Autodesk Inventor part; units mm, degrees
ref_plane "YZ Plane" through (0, 0, 0) normal (1, 0, 0) x (0, 1, 0)
ref_plane "XZ Plane" through (0, 0, 0) normal (0, 1, 0) x (-1, 0, 0)
ref_plane "XY Plane" through (0, 0, 0) normal (0, 0, 1) x (1, 0, 0)
sketch "Sketch1" plane through (0, 0, 0) normal (0, 0, 1) x (1, 0, 0)
  line L0 (0, 0) -> (25.7, 0)
  line L1 (25.7, 0) -> (25.7, 44.3)
  line L2 (25.7, 44.3) -> (0, 44.3)
  line L3 (0, 44.3) -> (0, 0)
  dimension "d0" = 25.7
  dimension "d1" = 44.3
extrude "Extrusion1" add sketch "Sketch1" along normal blind 16.6
sketch "Sketch2" plane through (0, 44.3, 0) normal (0, 1, 0) x (1, 0, 0)
  line L0 (0, 0) -> (0, -16.6)
  circle A0 centre (6.15, -8.3) radius 4.15
  circle A1 centre (19.55, -8.3) radius 2.85
  dimension "d4" = 8.3
  dimension "d5" = 5.7
  dimension "d6" = 13.4
  dimension "d7" = 6.15
extrude "Extrusion2" add sketch "Sketch2" along normal blind 3.3
sketch "Sketch3" plane through (6.15, 47.6, 8.3) normal (0, 1, 0) x (1, 0, 0)
  circle A0 centre (0, 0) radius 4.15
  circle A1 centre (0, 0) radius 2.85
  point P0 (-6.15, 8.3)
  dimension "d10" = 5.7
extrude "Extrusion3" cut sketch "Sketch3" against normal blind 3 contours A1
fillet "Fillet1" radius 3 4 edges at (25.7, 22.15, 16.6) (25.7, 22.15, 0) (0, 22.15, 16.6) (0, 22.15, 0)
fillet "Fillet2" radius 1 16 edges at (12.85, 44.3, 16.6) (24.8213, 44.3, 15.7213) (25.7, 44.3, 8.3) (24.8213, 44.3, 0.8787) (12.85, 44.3, 0) (0.8787, 44.3, 0.8787) (0, 44.3, 8.3) (0.8787, 44.3, 15.7213) (12.85, 0, 16.6) (0.8787, 0, 15.7213) (0, 0, 8.3) (0.8787, 0, 0.8787) (12.85, 0, 0) (24.8213, 0, 0.8787) (25.7, 0, 8.3) (24.8213, 0, 15.7213)
properties part number "Battery9V"
Can you work these out from the model? Positions are in its coordinate system, mm. A direction names the side the tool comes from. Coordinates: 2 decimals unless noted, no trailing zeros. Order: outer loops, then holes, each group sorted by start corner. A loop starts at its lowest first (then second) coordinate and runs counter-clockwise, first axis right, second up.
1. If we section it at C-C (z = 8.3): Please give me the cut outline in (x, y), then the cut area to 3 significant figures.
2. Thinking about a two-plate mould opening in X: for faces 1 (the face through (25.415, 43.999, 8.374)), 2 (the face through (12.712, 0.301, 0.285)), 3 (the face through (13, 44.3, 8)), which applies, +X half, -X half, draft (parallel to the pull), parting line (faces both ways), or undercut?
3. For faces 4 (the face through (0.285, 0.301, 8.374)), 5 (the face through (5.779, 46.121, 5.474)), which set-ups out of +Z, -Z, +X, -X, +Y, -Y let a thin tool reach every point of the face, with its end or its side?
4. If we section it at B-B (y = 42): Please give me the cut outline in (x, z), then the cut area to 3 significant figures.
5. If we section it at D-D (x = 6.15): Please give me the cut outline in (y, z).
6. I need wall thicknesses on line 1 (X direction, y = 45.5, z = 8.3); line 2 (Z direction, x = 6.15, y = 46.2); line 3 (Y direction, x = 21, z = 15.5). Which ranges of each line are inside material? Lowest first, please.
7. If we section it at A-A (x = 19.55): Please give me the cut outline in (y, z).
Entries:
1. outline: (0, 1) arc R1 ccw to (1, 0) - (24.7, 0) arc R1 ccw to (25.7, 1) - (25.7, 43.3) arc R1 ccw to (24.7, 44.3) - (22.4, 44.3) - (22.4, 47.6) - (16.7, 47.6) - (16.7, 44.3) - (10.3, 44.3) - (10.3, 47.6) - (9, 47.6) - (9, 44.6) - (3.3, 44.6) - (3.3, 47.6) - (2, 47.6) - (2, 44.3) - (1, 44.3) arc R1 ccw to (0, 43.3) - close
1. area: 1,170 mm2
2. face 1: +X half
2. face 2: draft
2. face 3: undercut
3. face 4: +Z, -Z, -X, -Y
3. face 5: +Y
4. outline: (0, 3) arc R3 ccw to (3, 0) - (22.7, 0) arc R3 ccw to (25.7, 3) - (25.7, 13.6) arc R3 ccw to (22.7, 16.6) - (3, 16.6) arc R3 ccw to (0, 13.6) - close
4. area: 419 mm2
5. outline: (0, 1) arc R1 ccw to (1, 0) - (43.3, 0) arc R1 ccw to (44.3, 1) - (44.3, 4.15) - (47.6, 4.15) - (47.6, 5.45) - (44.6, 5.45) - (44.6, 11.15) - (47.6, 11.15) - (47.6, 12.45) - (44.3, 12.45) - (44.3, 15.6) arc R1 ccw to (43.3, 16.6) - (1, 16.6) arc R1 ccw to (0, 15.6) - close
6. line 1: x = 2 to 3.3, 9 to 10.3, 16.7 to 22.4
6. line 2: z = 4.15 to 5.45, 11.15 to 12.45
6. line 3: y = 0 to 44.3
7. outline: (0, 1) arc R1 ccw to (1, 0) - (43.3, 0) arc R1 ccw to (44.3, 1) - (44.3, 5.45) - (47.6, 5.45) - (47.6, 11.15) - (44.3, 11.15) - (44.3, 15.6) arc R1 ccw to (43.3, 16.6) - (1, 16.6) arc R1 ccw to (0, 15.6) - close
